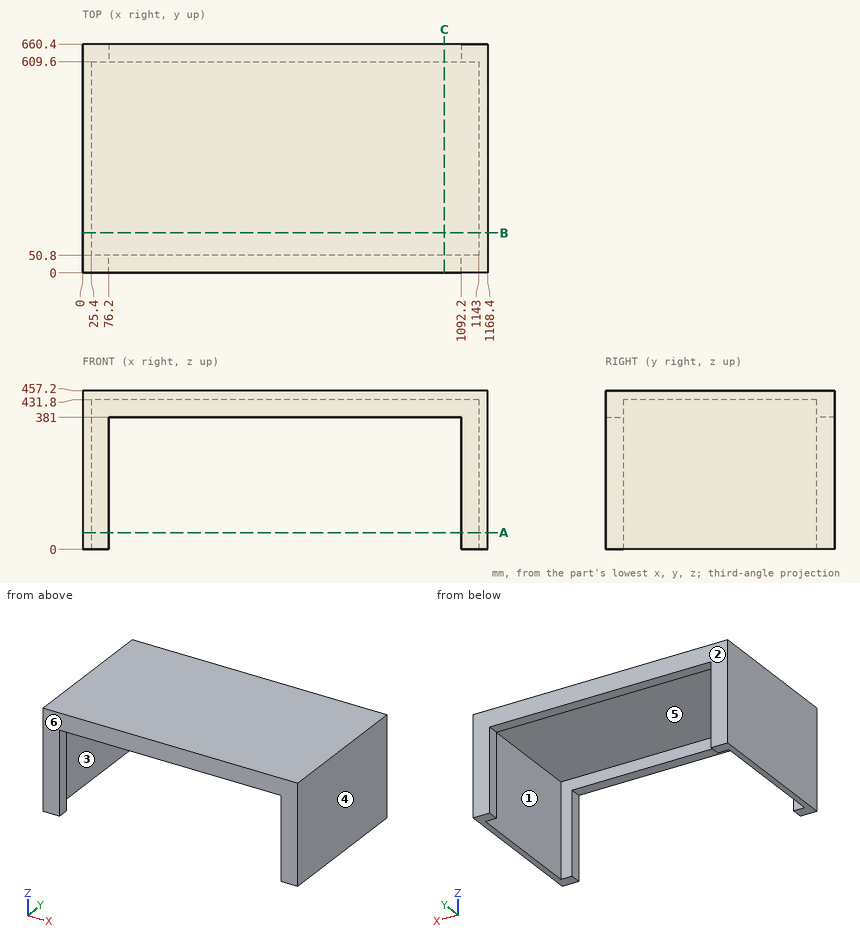
Geometry: see drawing. Coordinates: mm, zero at the bounding-box minimum. A direction names the side the tool comes from. Give positions to 0.01 mm unless a question says otherwise; leave off trailing zeros. Order: outer loops, then holes, each group sorted by start corner. A loop starts at its lowest first (then second) coordinate and runs counter-clockwise, first axis right, second up. Notation, with made-up numbers: (-13.5, 73.25) -> (11.5, 73.25) arc R24 cw to (11.5, 108.25) -> close; hole circle Ø9 at (64.5, 35). An arc over 180 degrees is marked (long way). Write item = value, one per line.
Q1. Pin query (flat end, axial travel): pin 1 (4 mm diameter, centred on x = 459, y = 480, fed in from -Z). Return the tip coordinate at first contact, or that it passes through.
Data:
pin_1 = 431.8
Q2. Material intervals for line 1 (X direction, y = 252, z = 162.5); line 2 (Y direction, x = 590, z = 426); line 3 (Z direction, x = 1092.5, y = 198.5), sorted ascending. Write a range as from..to.
Data:
line_1 = 0..25.4, 1143..1168.4
line_2 = 0..50.8, 609.6..660.4
line_3 = 431.8..457.2
Q3. Cut plane C-C, the plane x = 1043.5. Output: boundary loops of the cut face in (y, z), and give its area (3 significant figures).
Data:
outline = (0, 381) -> (50.8, 381) -> (50.8, 431.8) -> (609.6, 431.8) -> (609.6, 381) -> (660.4, 381) -> (660.4, 457.2) -> (0, 457.2) -> close
area = 21,900 mm^2
Q4. Cut plane B-B, the plane y = 115.5. Output: boundary loops of the cut face in (x, z), and give its area (3 significant figures).
Data:
outline = (0, 0) -> (25.4, 0) -> (25.4, 431.8) -> (1143, 431.8) -> (1143, 0) -> (1168.4, 0) -> (1168.4, 457.2) -> (0, 457.2) -> close
area = 51,600 mm^2
Q5. Cut plane A-A, the plane z = 48.5. Output: boundary loops of the cut face in (x, y), and give its area (3 significant figures).
Data:
outline = (0, 0) -> (76.2, 0) -> (76.2, 50.8) -> (25.4, 50.8) -> (25.4, 609.6) -> (76.2, 609.6) -> (76.2, 660.4) -> (0, 660.4) -> close; (1092.2, 0) -> (1168.4, 0) -> (1168.4, 660.4) -> (1092.2, 660.4) -> (1092.2, 609.6) -> (1143, 609.6) -> (1143, 50.8) -> (1092.2, 50.8) -> close
area = 43,900 mm^2
Q6. Set-up query: the marked faces 5 and 6. Return all of +Z, -Z, +X, -X, +Y, -Y with unobstructed straight access to the full face (end or side cutting, diameter ignored); none if empty.
Data:
face_5 = -Z
face_6 = +Z, -Z, +X, -X, -Y
Q7. Pull-direction query (X, two-part tool) for the marked faces 1, 2, 3 and 4; classes: released by +X, released by -X, zero draft, split by the parting line, or undercut.
Data:
face_1 = undercut
face_2 = zero draft
face_3 = undercut
face_4 = released by +X
